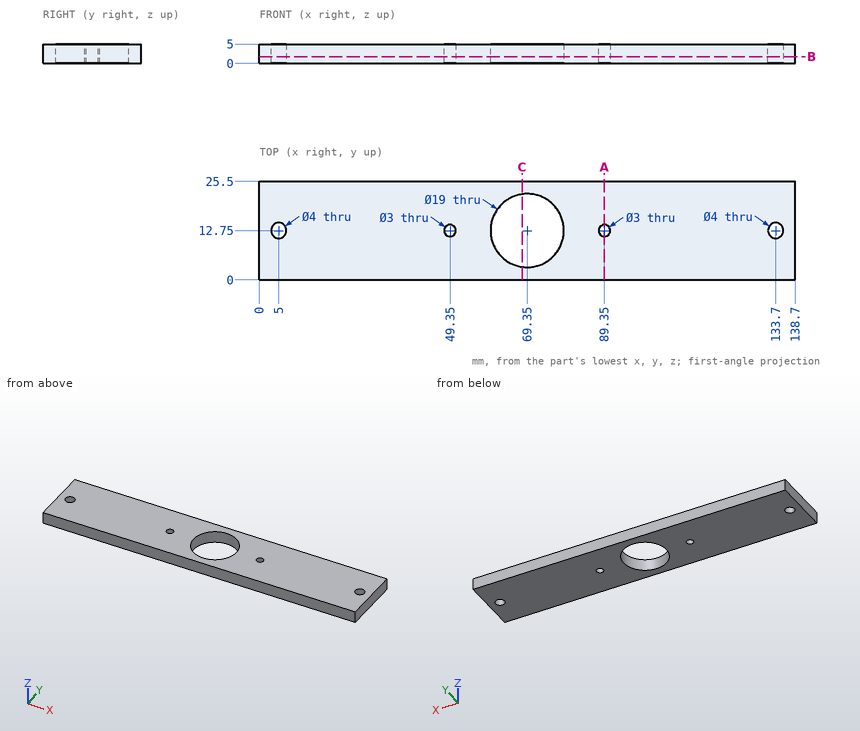
Source: three-view drawing plus pictorial views. Frame: mm from the lowest corner of the part. Round coordinates to 2 decimals unless told otherwise and drop trailing zeros. Write each loop counter-clockwise with the first axis right and the second up, starting at its lowest first coordinate (ties: lowest second). Pieces come first, ordered by that corner, then holes. Notation, with made-up numbers: M 50.5,82.5 L 71.5,82.5 A29 cw 71.5,110.5 Z; hole C -35,-30.75 d5. An arc over 180 degrees is marked long. Use CSV: the item, a comma, the result in double quotes. Start each with the question number.
Q1. Cut plane B-B on z = 1.75. Output: boundary loops of the cut face in (x, y).
Q2. Line query: line 1 (Y direction, x = 69.35, z = 3.95); line 2 (Y direction, x = 89.35, z = 3.45); line 3 (X direction, y = 8.75, z = 4.2). Output: solid intervals per line, ascending. Write a range as from..to.
Q3. Cut plane A-A on x = 89.35. Output: boundary loops of the cut face in (y, z), plus the area to 4 significant figures.
Q4. First-contact query: P1, Ø2.5, axis at x = 89.35, y = 12.75, coming from the +Z side; P2, Ø2, axis at y = 15.5, z = 2.5, coming from the -X side. Flat tips, straight axial feed; report the tip coordinate or a pass-through.
Q5. Cut plane C-C on x = 68. Output: boundary loops of the cut face in (y, z).
Results found:
1,outline,"M 0,0 L 138.7,0 L 138.7,25.5 L 0,25.5 Z; hole C 5,12.75 d4; hole C 49.35,12.75 d3; hole C 69.35,12.75 d19; hole C 89.35,12.75 d3; hole C 133.7,12.75 d4"
2,line 1,"0..3.25, 22.25..25.5"
2,line 2,"0..11.25, 14.25..25.5"
2,line 3,"0..60.73, 77.97..138.7"
3,outline,"M 0,0 L 11.25,0 L 11.25,5 L 0,5 Z; M 14.25,0 L 25.5,0 L 25.5,5 L 14.25,5 Z"
3,area,"112.5 mm^2"
4,P1,"through"
4,P2,"x = 0"
5,outline,"M 0,0 L 3.35,0 L 3.35,5 L 0,5 Z; M 22.15,0 L 25.5,0 L 25.5,5 L 22.15,5 Z"
